Can you work these out from the model? Positions are in its coordinate system, mm. A direction names the side the tool comes from. Coordinates: 2 decimals unless noted, no trailing zeros. Loops run counter-clockwise (first coordinate to the right, second up) from the corner with the lowest first, then second, coordinate; pieces in that order, holes last.
Autodesk Inventor part; units mm, degrees
ref_plane "YZ Plane" through (0, 0, 0) normal (1, 0, 0) x (0, 1, 0)
ref_plane "XZ Plane" through (0, 0, 0) normal (0, 1, 0) x (-1, 0, 0)
ref_plane "XY Plane" through (0, 0, 0) normal (0, 0, 1) x (1, 0, 0)
sketch "Sketch1" plane through (0, 0, 0) normal (0, 0, 1) x (1, 0, 0)
  line L0 (0, 0.2366) -> (10, 0.2366)
  line L1 (10, 0.2366) -> (10, 30.2366)
  line L2 (10, 30.2366) -> (0, 30.2366)
  line L3 (0, 30.2366) -> (0, 0.2366)
  point P0 (0, 0)
  dimension "d0" = 10
  dimension "d1" = 30
extrude "Extrusion1" add sketch "Sketch1" along normal blind 1
sketch "Sketch2" plane through (0, 30.2366, 0) normal (0, 1, 0) x (1, 0, 0)
  line L0 (0, 0) -> (0, -1)
  line L1 (0, -0.5) -> (10, -0.5)
  line L2 (0, 0) -> (10, 0)
  line L3 (2.646, -1) -> (2.646, 0.5163)
  line L4 (6.9484, -1) -> (6.9484, 0)
  circle A0 centre (2.646, -0.5) radius 0.5
  circle A1 centre (6.9484, -0.5) radius 0.5
  dimension "d4" = 1
extrude "Extrusion2" add sketch "Sketch2" along normal blind 2.5 contours A0 L1 L3 | L3 L1 A0 | L1 L3 A0 | A1 L1 L4 | L4 L1 A1 | L1 A0 L3 | L4 A1 L1 | L1 A1 L4
sketch "Sketch3" plane through (0, 0, 0) normal (0, 0, -1) x (-1, 0, 0)
  line L0 (-3.175, 1.5875) -> (-3.175, -3.4125)
  line L1 (-5, 1.5875) -> (-5, -3.4125)
  line L2 (-7.0347, 1.5875) -> (-7.0347, -3.4125)
  point P0 (0, 0)
  dimension "d7" = 5
  dimension "d8" = 5
  dimension "d9" = 5
sketch "Sketch4" plane through (0, 0, 1) normal (0, 0, 1) x (1, 0, 0)
  line L0 (4.7625, 30.1625) -> (4.7625, 25.1625)
  circle A0 centre (4.7625, 25.1625) radius 0.05
  point P0 (0, 0)
  dimension "d10" = 5
  dimension "d11" = 0.1
extrude "Extrusion3" cut sketch "Sketch4" against normal through all
properties part number "ir sensor"
Item 1: On a 3-axis mill with a long thin cutter (end or side, diameter ignored), from which of +Z, -Z, +X, -X, +Y, -Y can I reach the whole of each face in a straight line? I mean faces 1 (the face through (3.11, 31.47, 0.31)), 2 (the face through (5, 15, 1)). Say none if no direction works.
Results are:
face 1: +Y
face 2: +Z, +X, -X, +Y, -Y
Item 2: Suppose I cut it at B-B, the plane x = 5.25. Please give me the cut outline in (y, z), plus the area to 3 significant figures.
Results are:
outline: (0.24, 0) - (30.24, 0) - (30.24, 1) - (0.24, 1) - close
area: 30.0 mm2
Item 3: I need wall thicknesses on line 1 along Y through (x, z) = (5.25, 0.9). Which ranges of the line are inside material? Lowest first, please.
Results are:
line 1: y = 0.24 to 30.24
Item 4: Suppose I cut it at A-A, the plane z = 0.2. Please give me the cut outline in (x, y).
Results are:
outline: (0, 0.24) - (10, 0.24) - (10, 30.24) - (7.35, 30.24) - (7.35, 32.74) - (6.55, 32.74) - (6.55, 30.24) - (3.05, 30.24) - (3.05, 32.74) - (2.25, 32.74) - (2.25, 30.24) - (0, 30.24) - close; hole circle Ø0.1 at (4.76, 25.16)
Item 5: We'd pull the mould along X, two halves only. Please class faces 3 (the face through (0, 15.4, 0.5)), 4 (the face through (1, 30.237, 0.5)), 5 (the face through (4.8, 30.237, 0.5)): +X half, -X half, draft (parallel to the pull), parting line (faces both ways), or undercut.
Results are:
face 3: -X half
face 4: draft
face 5: undercut
